Verification items for the finished model (mm, model axes). A direction names the side the tool comes from. Round coordinates to 2 decimals unless told otherwise and drop trailing zeros. Order: outer loops, then holes, each group sorted by start corner. A loop starts at its lowest first (then second) coordinate and runs counter-clockwise, first axis right, second up. Notation, with made-up numbers: (1, 42.25) -> (49, 42.25) arc R20 cw to (49, 69.25) -> close; hole circle Ø7 at (-38, -10). An arc over 180 degrees is marked (long way). Return JSON: item names as keys, results as strings. Group by question number.
Item 1: Draft check along Z on faces 1 (the flat face through (-59.83, 0.04, 103.06)), 2 (the flat face through (-112.074, 0.042, 96.222)), 3 (the flat face through (-47.16, 0.04, 121.88)), 4 (the flat face through (27.983, 0.042, -144.772)). Enter one of: pulls with the +Z half, pulls with the -Z half, needs draft (parallel to the pull), parting line crosses it, or undercut.
Item 2: Sectioned sample at A-A on z = 57. Record the cut outline in (x, y).
Item 3: Depth check by flat-ended pin: pin 1 Ø1.5 at (x, y) = (96.5, 1.5) entering from -Z; pin 2 Ø2 at (x, y) = (80.5, -1.5) entering from -Z. Enter the tip coordinate at first touch or a pass-through.
Item 4: Sectioned sample at C-C on y = 1.4. Give the number of separate pieces and of enclosed holes in the cut face, plus the area to 3 significant figures.
Item 5: Sectioned sample at B-B on x = -94. Record the cut outline in (y, z), plus the area to 3 significant figures.
Item 6: Scan lines: probe 1 along X at (y, z) = (-1.4, -41.5); probe 2 along Z at (x, y) = (-106, -2.65); probe 3 along Z at (x, y) = (-7, 0.4). Record each from-to range of solid material in increasing order. Write a range as from..to.
Item 7: Access from +Z, -Z, +X, -X, +Y, -Y to the whole of each face (thin tool, end or side, straight path). Record for faces 5 (the flat face through (81.97, 0.04, 101.78)), 6 (the cylindrical face through (-102.012, 0.042, 64.445)), 7 (the flat face through (82.1, 0, -102)).
```python
from build123d import *

# Parameters (mm, degrees)
SKETCH1_R           = 1.45
BOSS_EXTRUDE2_DEPTH = 3
SKETCH2_R           = 1.45
CUT_EXTRUDE1_DEPTH  = 161.808628333
CIRPATTERN7_COUNT   = 6
SKETCH3_R           = 1.45
CUT_EXTRUDE2_DEPTH  = 213.272030532
SKETCH4_R           = 1.25
CUT_EXTRUDE3_DEPTH  = 213.272030532
SKETCH5_R           = 1.45
CUT_EXTRUDE4_DEPTH  = 213.272030532
SKETCH6_R           = 1.375
CUT_EXTRUDE5_DEPTH  = 213.272030532
SKETCH7_R           = 1.45
CUT_EXTRUDE6_DEPTH  = 213.272030532
SKETCH9_R           = 12.5
CUT_EXTRUDE7_DEPTH  = 213.272030532
SKETCH10_R          = 12.5
CUT_EXTRUDE8_DEPTH  = 213.272030532


with BuildPart() as part:
    # Sketch1 → Boss-Extrude2 (new, symmetric)
    with BuildSketch(Plane(origin=(0, 0, 0), x_dir=(1, 0, 0), z_dir=(0, 1, 0))):
        with BuildLine():
            Line((-139.367912183, 20.1), (-119.167912183, 20.1))
            Line((-119.167912183, 20.1), (-119.167912183, -20.1))
            Line((-119.167912183, -20.1), (-139.367912183, -20.1))
            Line((-139.367912183, -20.1), (-139.367912183, -77))
            ThreePointArc((-139.367912183, -77), (-139.163467141, -78.552914271), (-138.564064606, -80))
            Line((-138.564064606, -80), (0, 0))
            Line((0, 0), (-138.564064606, 80))
            ThreePointArc((-138.564064606, 80), (-139.163467141, 78.552914271), (-139.367912183, 77))
            Line((-139.367912183, 77), (-139.367912183, 20.1))
        make_face()
        with Locations(Location((-123.74355653, 65.669872981, 0), (0, 0, 270))):
            Circle(SKETCH1_R, mode=Mode.SUBTRACT)
        with Locations(Location((-123.74355653, -65.669872981, 0), (0, 0, 90))):
            Circle(SKETCH1_R, mode=Mode.SUBTRACT)
    boss_extrude2 = extrude(amount=BOSS_EXTRUDE2_DEPTH, both=True)

    # Sketch2 → Cut-Extrude1 (cut, through all)
    with BuildSketch(Plane(origin=(0, 3, 0), x_dir=(1, 0, 0), z_dir=(0, 1, 0))):
        with Locations(Location((-134.267912183, 24.8, 0), (0, 0, 270))):
            Circle(SKETCH2_R)
        with Locations(Location((-124.267912183, 24.8, 0), (0, 0, 90))):
            Circle(SKETCH2_R)
        with Locations(Location((-124.267912183, -24.8, 0), (0, 0, 270))):
            Circle(SKETCH2_R)
        with Locations(Location((-134.267912183, -24.8, 0), (0, 0, 90))):
            Circle(SKETCH2_R)
        with Locations(Location((-108.067912183, 15, 0), (0, 0, 270))):
            Circle(SKETCH2_R)
        with Locations(Location((-108.067912183, 5, 0), (0, 0, 270))):
            Circle(SKETCH2_R)
    cut_extrude1 = extrude(amount=-CUT_EXTRUDE1_DEPTH, mode=Mode.SUBTRACT)

    # CirPattern7: Boss-Extrude2, Cut-Extrude1 ×6 about axis
    cirpattern7_axis = Axis((0, 0, 0), (0, 1, 0))
    add([boss_extrude2.rotate(cirpattern7_axis, i * 360 / CIRPATTERN7_COUNT) for i in range(1, CIRPATTERN7_COUNT)])
    add([cut_extrude1.rotate(cirpattern7_axis, i * 360 / CIRPATTERN7_COUNT) for i in range(1, CIRPATTERN7_COUNT)], mode=Mode.SUBTRACT)

    # Sketch3 → Cut-Extrude2 (cut, through all)
    with BuildSketch(Plane(origin=(0, 3, 0), x_dir=(1, 0, 0), z_dir=(0, 1, 0))):
        with Locations(Location((-24.675, 24.675, 0), (0, 0, 270))):
            Circle(SKETCH3_R)
        with Locations(Location((24.675, 24.675, 0), (0, 0, 90))):
            Circle(SKETCH3_R)
        with Locations(Location((24.675, -24.675, 0), (0, 0, 270))):
            Circle(SKETCH3_R)
        with Locations(Location((-24.675, -24.675, 0), (0, 0, 90))):
            Circle(SKETCH3_R)
    extrude(amount=-CUT_EXTRUDE2_DEPTH, mode=Mode.SUBTRACT)

    # Sketch4 → Cut-Extrude3 (cut, through all)
    with BuildSketch(Plane(origin=(0, 3, 0), x_dir=(1, 0, 0), z_dir=(0, 1, 0))):
        with Locations(Location((38, 27.95, 0), (0, 0, 270))):
            Circle(SKETCH4_R)
        with Locations(Location((56.8, 27.95, 0), (0, 0, 270))):
            Circle(SKETCH4_R)
        with Locations(Location((68.1, 27.95, 0), (0, 0, 270))):
            Circle(SKETCH4_R)
        with Locations(Location((86.9, 27.95, 0), (0, 0, 270))):
            Circle(SKETCH4_R)
        with Locations(Location((86.9, -27.95, 0), (0, 0, 90))):
            Circle(SKETCH4_R)
        with Locations(Location((68.1, -27.95, 0), (0, 0, 90))):
            Circle(SKETCH4_R)
        with Locations(Location((56.8, -27.95, 0), (0, 0, 90))):
            Circle(SKETCH4_R)
        with Locations(Location((38, -27.95, 0), (0, 0, 90))):
            Circle(SKETCH4_R)
    extrude(amount=-CUT_EXTRUDE3_DEPTH, mode=Mode.SUBTRACT)

    # Sketch5 → Cut-Extrude4 (cut, through all)
    with BuildSketch(Plane(origin=(0, 3, 0), x_dir=(1, 0, 0), z_dir=(0, 1, 0))):
        with Locations(Location((-85.46, -35.53, 0), (0, 0, 270))):
            Circle(SKETCH5_R)
        with Locations(Location((-85.46, 39.35, 0), (0, 0, 270))):
            Circle(SKETCH5_R)
        with Locations(Location((-37.24, 45.71, 0), (0, 0, 270))):
            Circle(SKETCH5_R)
        with Locations(Location((-37.24, -36.76, 0), (0, 0, 270))):
            Circle(SKETCH5_R)
    extrude(amount=-CUT_EXTRUDE4_DEPTH, mode=Mode.SUBTRACT)

    # Sketch6 → Cut-Extrude5 (cut, through all)
    with BuildSketch(Plane(origin=(0, 3, 0), x_dir=(1, 0, 0), z_dir=(0, 1, 0))):
        with Locations(Location((-26.5, -39.45, 0), (0, 0, 270))):
            Circle(SKETCH6_R)
        with Locations(Location((31.5, -39.45, 0), (0, 0, 270))):
            Circle(SKETCH6_R)
        with Locations(Location((31.5, -88.45, 0), (0, 0, 270))):
            Circle(SKETCH6_R)
        with Locations(Location((-26.5, -88.45, 0), (0, 0, 270))):
            Circle(SKETCH6_R)
    extrude(amount=-CUT_EXTRUDE5_DEPTH, mode=Mode.SUBTRACT)

    # Sketch7 → Cut-Extrude6 (cut, through all)
    with BuildSketch(Plane(origin=(0, 3, 0), x_dir=(1, 0, 0), z_dir=(0, 1, 0))):
        with Locations(Location((-26.415, 78.025, 0), (0, 0, 270))):
            Circle(SKETCH7_R)
        with Locations(Location((26.415, 78.025, 0), (0, 0, 270))):
            Circle(SKETCH7_R)
        with Locations(Location((26.415, 41.395, 0), (0, 0, 270))):
            Circle(SKETCH7_R)
        with Locations(Location((-26.415, 41.395, 0), (0, 0, 270))):
            Circle(SKETCH7_R)
    extrude(amount=-CUT_EXTRUDE6_DEPTH, mode=Mode.SUBTRACT)

    # Sketch9 → Cut-Extrude7 (cut, through all)
    with BuildSketch(Plane(origin=(0, 3, 0), x_dir=(1, 0, 0), z_dir=(0, 1, 0))):
        with Locations(Location((89.419235407, -51.626219633, 0), (0, 0, 270))):
            Circle(SKETCH9_R)
        with Locations(Location((89.419235407, 51.626219633, 0), (0, 0, 90))):
            Circle(SKETCH9_R)
        with BuildLine():
            Line((-108, -29.76), (-108, -49.76))
            ThreePointArc((-108, -49.76), (-101.849242405, -64.609242405), (-87, -70.76))
            Line((-87, -70.76), (-44.5, -70.76))
            ThreePointArc((-44.5, -70.76), (-39.5, -65.76), (-44.5, -60.76))
            Line((-44.5, -60.76), (-87, -60.76))
            ThreePointArc((-87, -60.76), (-94.778174593, -57.538174593), (-98, -49.76))
            Line((-98, -49.76), (-98, -29.76))
            ThreePointArc((-98, -29.76), (-103, -24.76), (-108, -29.76))
        make_face()
        with BuildLine():
            Line((-98, 49.76), (-98, 29.76))
            ThreePointArc((-98, 29.76), (-103, 24.76), (-108, 29.76))
            Line((-108, 29.76), (-108, 49.76))
            ThreePointArc((-108, 49.76), (-101.849242405, 64.609242405), (-87, 70.76))
            Line((-87, 70.76), (-44.5, 70.76))
            ThreePointArc((-44.5, 70.76), (-39.5, 65.76), (-44.5, 60.76))
            Line((-44.5, 60.76), (-87, 60.76))
            ThreePointArc((-87, 60.76), (-94.778174593, 57.538174593), (-98, 49.76))
        make_face()
    extrude(amount=-CUT_EXTRUDE7_DEPTH, mode=Mode.SUBTRACT)

    # Sketch10 → Cut-Extrude8 (cut, through all)
    with BuildSketch(Plane(origin=(0, 3, 0), x_dir=(1, 0, 0), z_dir=(0, 1, 0))):
        with Locations(Location((0, -113.252439266, 0), (0, 0, 270))):
            Circle(SKETCH10_R)
        with Locations(Location((0, 113.252439266, 0), (0, 0, 90))):
            Circle(SKETCH10_R)
    extrude(amount=-CUT_EXTRUDE8_DEPTH, mode=Mode.SUBTRACT)


solid = part.part
```
Recorded:
{
 "1": {"face 1": "undercut", "face 2": "pulls with the +Z half", "face 3": "undercut", "face 4": "pulls with the -Z half"},
 "2": {"outline": "(-139.37, -3) -> (-106.71, -3) -> (-106.71, 3) -> (-139.37, 3) -> close; (-95.28, -3) -> (78.13, -3) -> (78.13, 3) -> (-95.28, 3) -> close; (100.71, -3) -> (139.37, -3) -> (139.37, 3) -> (100.71, 3) -> close"},
 "3": {"pin 1": "z = -105.65", "pin 2": "z = -100.96"},
 "4": {"separate pieces": "1", "enclosed holes": "78", "area": "58,100 mm²"},
 "5": {"outline": "(-3, -106.66) -> (3, -106.66) -> (3, -69.56) -> (-3, -69.56) -> close; (-3, -58.25) -> (3, -58.25) -> (3, 58.25) -> (-3, 58.25) -> close; (-3, 69.56) -> (3, 69.56) -> (3, 106.66) -> (-3, 106.66) -> close", "area": "1,140 mm²"},
 "6": {"probe 1": "-139.37..-108, -98..-27.86, -24.97..24.97, 27.86..82.09, 96.75..139.37", "probe 2": "-99.73..-58.7, -25.76..25.76, 58.7..99.73", "probe 3": "-156.89..-123.61, -102.9..102.9, 123.61..156.89"},
 "7": {"face 5": "+Z, +Y, -Y", "face 6": "+Y, -Y", "face 7": "-Z, +Y, -Y"}
}
